```python
from build123d import *

# Parameters (mm, degrees)
F0_W      = 30
F0_H      = 25
F1_DEPTH  = 17
F3_DEPTH  = 11
F4_R      = 3.75
F5_DEPTH  = 25
F7_DEPTH  = 12
F9_DEPTH  = 12
F10_R     = 1.8
F11_DEPTH = 8.5
F12_R     = 1.8
F13_DEPTH = 2.6
F15_DEPTH = 8
F16_R     = 1.8
F17_DEPTH = 14
F18_R     = 1.8
F19_DEPTH = 2.5
F21_SIZE  = 0.5
F22_SIZE2 = 1
F22_SIZE  = 1
F23_R     = 1.35
F24_DEPTH = 5.0024289631


with BuildPart() as f1:
    # F0 (on Top) → F1 (new body)
    with BuildSketch(Plane.XY):
        Rectangle(F0_W, F0_H)
    extrude(amount=F1_DEPTH)

    # F2 (on face) → F3 (cut)
    with BuildSketch(Plane.XZ.offset(12.5)):
        Polygon((10, 17), (2, 17), (2, 3.5), (12, 3.5), (12, 11.5), (10, 13.5), align=None)
    extrude(amount=-F3_DEPTH, mode=Mode.SUBTRACT)

    # F4 (on face) → F5 (cut, through all)
    with BuildSketch(Plane.XZ.offset(12.5)):
        with Locations((-6.5, 8.5)):
            Circle(F4_R)
    extrude(amount=-F5_DEPTH, mode=Mode.SUBTRACT)

    # F6 (on face) → F7 (join)
    with BuildSketch(Plane.XY.offset(17)):
        Polygon((-6.5, -12.5), (2, -12.5), (2, -1.5), (2, 12.5), (-6.5, 12.5), align=None)
    extrude(amount=F7_DEPTH)

    # F8 (on face) → F9 (cut)
    with BuildSketch(Plane.XY.offset(29)):
        with BuildLine():
            Line((-6.5, 4.1892720131), (-6.5, -4.1892720131))
            ThreePointArc((-6.5, -4.1892720131), (-2.6, 0), (-6.5, 4.1892720131))
        make_face()
    extrude(amount=-F9_DEPTH, mode=Mode.SUBTRACT)

    # F10 (on face) → F11 (cut, through all)
    with BuildSketch(Plane(origin=(-6.5, 0, 0), x_dir=(0, -1, 0), z_dir=(-1, 0, 0))):
        with Locations((-8.3446360066, 23)):
            Circle(F10_R)
        with Locations((8.3446360066, 23)):
            Circle(F10_R)
    extrude(amount=-F11_DEPTH, mode=Mode.SUBTRACT)

    # F12 (on face) → F13 (cut)
    with BuildSketch(Plane.YZ.offset(2)):
        Polygon((11.3446360067, 21.2679491924), (11.3446360067, 24.7320508076), (8.3446360067, 26.4641016151), (5.3446360067, 24.7320508076), (5.3446360067, 21.2679491924), (8.3446360067, 19.5358983849), align=None)
        with Locations((8.3446360066, 23)):
            Circle(F12_R, mode=Mode.SUBTRACT)
        Polygon((-5.3446360065, 21.2679491924), (-5.3446360065, 24.7320508076), (-8.3446360065, 26.4641016151), (-11.3446360065, 24.7320508076), (-11.3446360065, 21.2679491924), (-8.3446360065, 19.5358983849), align=None)
        with Locations((-8.3446360066, 23)):
            Circle(F12_R, mode=Mode.SUBTRACT)
    extrude(amount=-F13_DEPTH, mode=Mode.SUBTRACT)

    # F14 (on face) → F15 (cut)
    with BuildSketch(Plane.XY.offset(17)):
        with BuildLine():
            Line((5.95, 12.5), (4.5, 12.5))
            Line((4.5, 12.5), (4.5, 3.5))
            Line((4.5, 3.5), (5.95, 3.5))
            Line((5.95, 3.5), (5.95, 4.9))
            ThreePointArc((5.95, 4.9), (5.35, 5.5), (5.95, 6.1))
            Line((5.95, 6.1), (5.95, 6.9))
            ThreePointArc((5.95, 6.9), (5.35, 7.5), (5.95, 8.1))
            Line((5.95, 8.1), (5.95, 8.9))
            ThreePointArc((5.95, 8.9), (5.35, 9.5), (5.95, 10.1))
            Line((5.95, 10.1), (5.95, 10.9))
            ThreePointArc((5.95, 10.9), (5.35, 11.5), (5.95, 12.1))
            Line((5.95, 12.1), (5.95, 12.5))
        make_face()
    extrude(amount=-F15_DEPTH, mode=Mode.SUBTRACT)

    # F16 (on face) → F17 (cut, through all)
    with BuildSketch(Plane(origin=(0, 12.5, 0), x_dir=(-1, 0, 0), z_dir=(0, 1, 0))):
        with Locations((-9.05, 6.5)):
            Circle(F16_R)
    extrude(amount=-F17_DEPTH, mode=Mode.SUBTRACT)

    # F18 (on face) → F19 (cut)
    with BuildSketch(Plane(origin=(0, 12.5, 0), x_dir=(-1, 0, 0), z_dir=(0, 1, 0))):
        Polygon((-7.3179491924, 9.5), (-10.7820508076, 9.5), (-12.5141016151, 6.5), (-10.7820508076, 3.5), (-7.3179491924, 3.5), (-5.5858983849, 6.5), align=None)
        with Locations((-9.05, 6.5)):
            Circle(F18_R, mode=Mode.SUBTRACT)
    extrude(amount=-F19_DEPTH, mode=Mode.SUBTRACT)

    # F21
    f21_edges = [f1.edges().sort_by_distance(p)[0] for p in [
        (0, -12.5, 0),
        (-15, 0, 0),
        (0, 12.5, 0),
        (15, 0, 0),
        (-15, 0, 17),
        (-10.75, 12.5, 17),
        (-15, 12.5, 8.5),
        (-15, -12.5, 8.5),
        (2, -12.5, 16.25),
        (7, -12.5, 3.5),
        (12, -12.5, 7.5),
        (11, -12.5, 12.5),
        (10, -12.5, 15.25),
        (15, -12.5, 8.5),
        (12.5, -12.5, 17),
        (15, 0, 17),
        (15, 12.5, 8.5),
        (10.475, 12.5, 17),
        (3.25, 12.5, 17),
        (2, 12.5, 23),
        (-6.5, 12.5, 23),
        (-2.25, 12.5, 29),
        (2, 0, 29),
        (-2.25, -12.5, 29),
        (-10.75, -12.5, 17),
        (-6.5, -8.344636, 29),
        (-2.6, 0, 29),
        (-6.5, 8.344636, 29),
    ]]
    chamfer(f21_edges, length=F21_SIZE)

    # F22
    f22_edges = [f1.edges().sort_by_distance(p)[0] for p in [
        (-2.75, 0, 8.5),
        (-10.25, -12.5, 8.5),
        (-10.25, 12.5, 8.5),
    ]]
    chamfer(f22_edges, length=F22_SIZE, length2=F22_SIZE2)

    # F23 (on face) → F24 (cut, through all)
    with BuildSketch(Plane(origin=(-15, 0, 0), x_dir=(0, -1, 0), z_dir=(-1, 0, 0))):
        with Locations((0, 8.5)):
            Circle(F23_R)
    extrude(amount=-F24_DEPTH, mode=Mode.SUBTRACT)


solid = f1.part
```
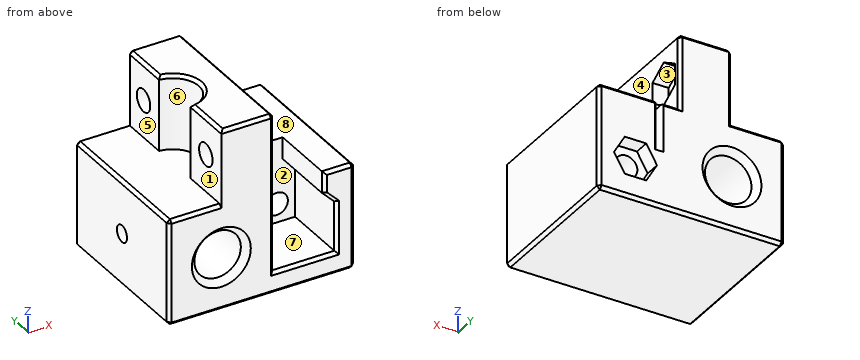
Can you work these out from the model? Positions are in its coordinate system, mm. Face numbers are marked on the shaded views. A direction names the side the tool comes from. Round coordinates to 2 decimals unless told otherwise and drop trailing zeros. Loops run counter-clockwise (first coordinate to the right, second up) from the corner with the lowest first, then second, coordinate; pieces in that order, holes last. Notation, with made-up numbers: (67.5, -17.5) -> (107.5, -17.5) arc R29 cw to (107.5, 18.5) -> close; hole circle Ø6 at (-34, -35.5). An arc over 180 degrees is marked (long way). One line per item, written item: value. Start each with the question number.
1. For the marked faces 4, 5, 6, 7 and 8, which set-ups out of +Z, -Z, +X, -X, +Y, -Y let a thin tool reach every point of the face, with its end or its side?
2. For pin 1 (4.5 mm diameter, centred on y = 8.34, z = 23, fed in from +X); pin 2 (0.8 mm diameter, centred on x = 9.5, y = 11.5, fed in from +Z); pin 3 (5 mm diameter, centred on y = 9.5, z = 23.5, fed in from +X), each with a flat end and sliding along its axis, tell me the tip position at first contact or that it passes through.
3. If we mould it in two halves opening along Y, with no side actions, what happens to the marked faces 1, 2 and 3? For each: pulls with the +Y half, pulls with the -Y half, needs draft (parallel to the pull), parting line crosses it, or undercut.
4. If we section it at B-B, the plane y = 0: Write out the boundary of the cut face in (x, z).
5. If we section it at A-A, the plane x = 9.05: Write out the boundary of the cut face in (y, z).
6. If we section it at C-C, the plane y = 9.5: Write out the boundary of the cut face in (x, z), then the cut area to 3 significant figures.
7. If I drill on probe 1 along X at (y, z) = (-4.75, 8.5); probe 2 along Y at (x, z) = (-13.5, 8.5); probe 3 along X at (y, z) = (-10, 13.75), over which ranges is the centre line in solid material (lowest first)?
8. If we section it at D-D, the plane x = 4: Write out the boundary of the cut face in (y, z), then the cut area to 3 significant figures.
Calculated:
1. face 4: +Z, -Y
1. face 5: +Z, -X, +Y, -Y
1. face 6: +Z, -X
1. face 7: -Y
1. face 8: +Z, +X, +Y, -Y
2. pin 1: stops at x = -0.6
2. pin 2: stops at z = 17
2. pin 3: stops at x = 2
3. face 1: needs draft
3. face 2: pulls with the -Y half
3. face 3: undercut
4. outline: (-15, 0.5) -> (-14.5, 0) -> (14.5, 0) -> (15, 0.5) -> (15, 16.5) -> (14.5, 17) -> (2, 17) -> (2, 28.5) -> (1.5, 29) -> (-2.1, 29) -> (-2.6, 28.5) -> (-2.6, 17) -> (-14.5, 17) -> (-15, 16.5) -> (-15, 9.85) -> (-10, 9.85) arc R3.75 cw (long way) to (-10, 7.15) -> (-15, 7.15) -> close; hole circle Ø3.6 at (9.05, 6.5)
5. outline: (-12.5, 0.5) -> (-12, 0) -> (12, 0) -> (12.5, 0.5) -> (12.5, 3.5) -> (10, 3.5) -> (10, 4.7) -> (-1.5, 4.7) -> (-1.5, 3.5) -> (-12, 3.5) -> (-12.5, 3) -> close; (-1.5, 8.3) -> (10, 8.3) -> (10, 9.5) -> (12.5, 9.5) -> (12.5, 16.5) -> (12, 17) -> (-1.5, 17) -> close
6. outline: (-15, 0.5) -> (-14.5, 0) -> (14.5, 0) -> (15, 0.5) -> (15, 16.5) -> (14.5, 17) -> (5.35, 17) -> (5.35, 9) -> (4.5, 9) -> (4.5, 17) -> (2, 17) -> (2, 20.2) -> (-0.6, 20.2) -> (-0.6, 21.62) -> (-6.5, 21.62) -> (-6.5, 17) -> (-14.5, 17) -> (-15, 16.5) -> close; (-6.5, 24.38) -> (-0.6, 24.38) -> (-0.6, 25.8) -> (2, 25.8) -> (2, 28.5) -> (1.5, 29) -> (-6, 29) -> (-6.5, 28.5) -> close; hole circle Ø7.5 at (-6.5, 8.5); hole circle Ø3.6 at (9.05, 6.5)
6. area: 519 mm²
7. probe 1: x = -15 to -10.25, -2.75 to 2, 12 to 15
7. probe 2: y = -12.5 to -1.35, 1.35 to 12.5
7. probe 3: x = -15 to 2, 10 to 15
8. outline: (-12.5, 0.5) -> (-12, 0) -> (12, 0) -> (12.5, 0.5) -> (12.5, 16.5) -> (12, 17) -> (-1.5, 17) -> (-1.5, 3.5) -> (-12, 3.5) -> (-12.5, 3) -> close
8. area: 276 mm²
